Check sheet for the modelled part. Datum: model origin and axes. Units: mm. Face numbers are marked on the shaded views. A direction names the side the tool comes from. Round coordinates to 2 decimals unless told otherwise and drop trailing zeros. Write each loop counter-clockwise with the first axis right and the second up, starting at its lowest first coordinate (ties: lowest second). Pieces come first, ordered by that corner, then holes. Notation, with made-up numbers: (57.5, 1) -> (111.5, 1) arc R16 ccw to (111.5, 6) -> close; hole circle Ø8 at (72, -40). An arc over 180 degrees is marked (long way). One line per item, written item: value.
Solid Edge part; units mm, degrees
sketch "Sketch1" plane through (0, 0, 0) normal (0, -1, 0) x (1, 0, 0)
  line L0 (-3, 40.4) -> (101, 40.4)
  line L1 (101, 40.4) -> (101, 0)
  line L2 (98, 0) -> (101, 0)
  line L3 (98, 37.4) -> (98, 0)
  line L4 (0, 37.4) -> (98, 37.4)
  line L5 (0, 0) -> (0, 37.4)
  line L6 (0, 0) -> (-3, 0)
  line L7 (-3, 0) -> (-3, 40.4)
  line L8 (-3, 3) -> (-15, 3)
  line L9 (-15, 3) -> (-15, 0)
  line L10 (-15, 0) -> (-3, 0)
  line L11 (-3, 0) -> (-3, 3)
  line L12 (113, 3) -> (101, 3)
  line L13 (101, 3) -> (101, 0)
  line L14 (101, 0) -> (113, 0)
  line L15 (113, 0) -> (113, 3)
extrude "Protrusion1" add sketch "Sketch1" against normal blind 12
fillet "Redondeo_1" radius 6 4 edges at (113, 0, 1.5) (113, 12, 1.5) (-15, 0, 1.5) (-15, 12, 1.5)
sketch "Sketch2" plane through (-7.5, 6, 0) normal (0, 0, -1) x (1, 0, 0)
  circle A0 centre (-1.5, 0) radius 2
  circle A1 centre (114.5, 0) radius 2
extrude "Cutout1" cut sketch "Sketch2" against normal up to next
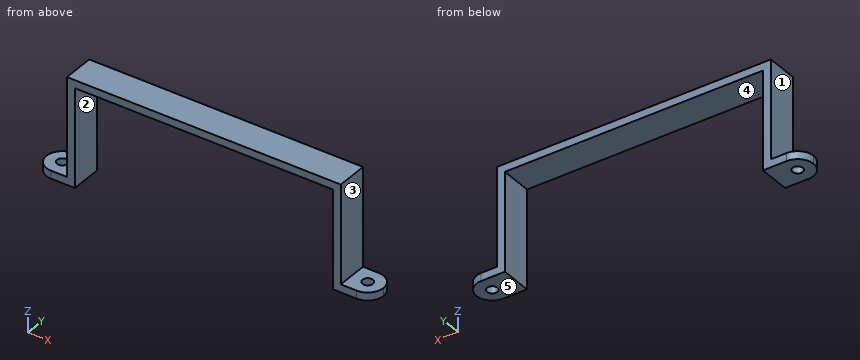
Item 1: Tool access check on the marked faces 4 and 5. Record the directions out of +Z, -Z, +X, -X, +Y, -Y that give a thin tool (end or side, any length) a straight path to the whole face; none if there is none.
Answer:
face 4: -Z, +Y, -Y
face 5: -Z, +X, -X, +Y, -Y
Item 2: Thickness scan on line 1 (X direction, y = 6, z = 1.5); line 2 (Y direction, x = 107, z = 1.05); line 3 (X direction, y = 3.25, z = 19). Record the ranges inside material, lowest first.
Answer:
line 1: x = -15 to -11, -7 to 0, 98 to 105, 109 to 113
line 2: y = 0 to 4, 8 to 12
line 3: x = -3 to 0, 98 to 101
Item 3: Depth check by flat-ended pin: P1, Ø5, axis at x = 45.5, y = 6.5, coming from the -Z side; P2, Ø6, axis at y = 8, z = 34.5, coming from the -X side; P3, Ø3.5, axis at x = 108, y = 6, coming from the +Z side. Enter the tip coordinate at first touch or a pass-through.
Answer:
P1: stops at z = 37.4
P2: stops at x = -3
P3: stops at z = 3
Item 4: Sectioned sample at B-B on x = 45. Enter the section's corners in (y, z).
Answer:
outline: (0, 37.4) -> (12, 37.4) -> (12, 40.4) -> (0, 40.4) -> close
Item 5: Mould release check, pull along X, two halves, no side actions. Record for the marked faces 1, 2 and 3: pulls with the +X half, pulls with the -X half, needs draft (parallel to the pull), parting line crosses it, or undercut.
Answer:
face 1: pulls with the -X half
face 2: undercut
face 3: pulls with the +X half
Item 6: Sectioned sample at C-C on y = 2. Enter the section's corners in (x, z), and give its area (3 significant figures).
Answer:
outline: (-13.47, 0) -> (0, 0) -> (0, 37.4) -> (98, 37.4) -> (98, 0) -> (111.47, 0) -> (111.47, 3) -> (101, 3) -> (101, 40.4) -> (-3, 40.4) -> (-3, 3) -> (-13.47, 3) -> close
area: 599 mm^2
Item 7: Sectioned sample at A-A on z = 15.5. Enter the section's corners in (x, y), and give its area (3 significant figures).
Answer:
outline: (-3, 0) -> (0, 0) -> (0, 12) -> (-3, 12) -> close; (98, 0) -> (101, 0) -> (101, 12) -> (98, 12) -> close
area: 72.0 mm^2
